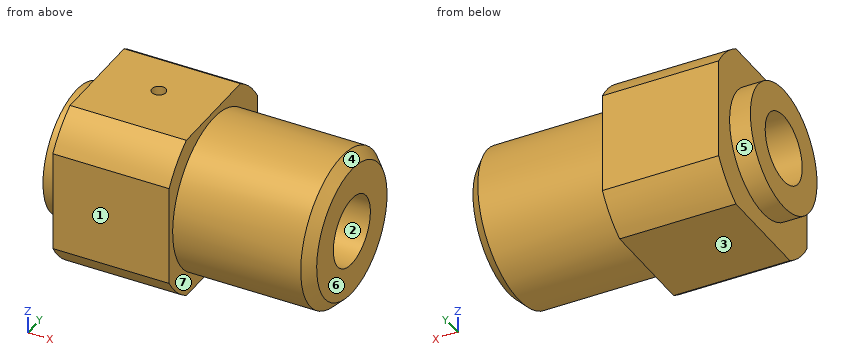
```python
from build123d import *

# Parameters (mm, degrees)
CROQUIS2_OUTSIDE_W      = 40.812
CROQUIS2_OUTSIDE_H      = 40.812
CROQUIS2_OUTSIDE_W_2    = 23.9
CROQUIS2_OUTSIDE_H_2    = 23.9
CORTAR_EXTRUIR1_DEPTH   = 42.788036566
CROQUIS4_R              = 5
CORTAR_EXTRUIR2_DEPTH   = 41.494999691
CROQUIS3_R              = 1
CORTAR_EXTRUIR3_DEPTH   = 13
CROQUIS5_R              = 9
CROQUIS5_R_2            = 5
SALIENTE_EXTRUIR1_DEPTH = 3


with BuildPart() as part:
    # Croquis1 → Revolución1 (revolve)
    with BuildSketch(Plane(origin=(0, 0, 0), x_dir=(1, 0, 0), z_dir=(0, 1, 0)), mode=Mode.PRIVATE) as revoluci_n1_sk:
        Polygon((0, 0), (36.8, 0), (36.8, 9.5), (35.3, 11), (16.8, 11), (16.8, 14), (0, 14), align=None)
    revolve(revoluci_n1_sk.sketch.rotate(Axis((0, 0, 0), (1, 0, 0)), 180), axis=Axis((0, 0, 0), (1, 0, 0)))

    # Croquis2 outside → Cortar-Extruir1 (cut, through all)
    with BuildSketch(Plane(origin=(0, 0, 0), x_dir=(0, 0, -1), z_dir=(1, 0, 0))):
        Rectangle(CROQUIS2_OUTSIDE_W, CROQUIS2_OUTSIDE_H)
        Rectangle(CROQUIS2_OUTSIDE_W_2, CROQUIS2_OUTSIDE_H_2, mode=Mode.SUBTRACT)
    extrude(amount=CORTAR_EXTRUIR1_DEPTH, mode=Mode.SUBTRACT)

    # Croquis4 → Cortar-Extruir2 (cut, through all)
    with BuildSketch(Plane(origin=(36.8, 0, 0), x_dir=(0, 0, -1), z_dir=(1, 0, 0))):
        Circle(CROQUIS4_R)
    extrude(amount=-CORTAR_EXTRUIR2_DEPTH, mode=Mode.SUBTRACT)

    # Croquis3 → Cortar-Extruir3 (cut)
    with BuildSketch(Plane.XY.offset(11.95)):
        with Locations((8.4, 0.993661632)):
            Circle(CROQUIS3_R)
    extrude(amount=-CORTAR_EXTRUIR3_DEPTH, mode=Mode.SUBTRACT)

    # Croquis5 → Saliente-Extruir1 (add)
    with BuildSketch(Plane.ZY):
        with Locations(Location((0, 0, 0), (0, 0, 180))):
            Circle(CROQUIS5_R)
        with Locations(Location((0, 0, 0), (0, 0, 180))):
            Circle(CROQUIS5_R_2, mode=Mode.SUBTRACT)
    extrude(amount=SALIENTE_EXTRUIR1_DEPTH)


solid = part.part
```
Design review of the part built by this model. Coordinates are the model's own, in mm. Face numbers are marked on the shaded views. A direction names the side the tool comes from. Coordinates: 2 decimals unless noted, no trailing zeros. Loops run counter-clockwise (first coordinate to the right, second up) from the corner with the lowest first, then second, coordinate; pieces in that order, holes last. Notation, with made-up numbers: (-16.75, -40) -> (5.25, -40) arc R31 ccw to (5.25, -3) -> close; hole circle Ø5 at (-37.5, 8). An arc over 180 degrees is marked (long way). Answer as a JSON object with one key per item and string values.
Q1. The part is to be moulded in two halves that separate along Y. For the marked faces 1, 2, 3 and 4, say which applies: +Y half, -Y half, draft (parallel to the pull), parting line (faces both ways), or undercut.
Answer block:
{"face 1": "-Y half", "face 2": "undercut", "face 3": "draft", "face 4": "parting line"}
Q2. Take a section at B-B on x = 8.4. Give the boundary of the cut face in (y, z), plus the area to 3 significant figures.
Answer block:
{"outline": "(-11.95, -7.29) arc R14 ccw to (-7.29, -11.95) -> (7.29, -11.95) arc R14 ccw to (11.95, -7.29) -> (11.95, 7.29) arc R14 ccw to (7.29, 11.95) -> (1.99, 11.95) -> (1.99, 4.59) arc R5 cw (long way) to (-0.01, 5) -> (-0.01, 11.95) -> (-7.29, 11.95) arc R14 ccw to (-11.95, 7.29) -> close", "area": "442 mm^2"}
Q3. Tool access review of the marked faces 5, 6 and 7: name each direction out of +Z, -Z, +X, -X, +Y, -Y from which nothing blocks a thin tool from reaching the whole face with its end or side.
Answer block:
{"face 5": "-X", "face 6": "+Z, -Z, +X, +Y, -Y", "face 7": "+X"}
Q4. Take a section at A-A on z = 0. Give the boundary of the cut face in (x, y), plus the area to 3 significant figures.
Answer block:
{"outline": "(-3, -9) -> (0, -9) -> (0, -11.95) -> (16.8, -11.95) -> (16.8, -11) -> (35.3, -11) -> (36.8, -9.5) -> (36.8, -5) -> (-3, -5) -> close; (-3, 5) -> (36.8, 5) -> (36.8, 9.5) -> (35.3, 11) -> (16.8, 11) -> (16.8, 11.95) -> (0, 11.95) -> (0, 9) -> (-3, 9) -> close", "area": "495 mm^2"}
Q5. Take a section at D-D on x = 26. Give the boundary of the cut face in (y, z).
Answer block:
{"outline": "circle Ø22 at (0, 0); hole circle Ø10 at (0, 0)"}
Q6. To check wall thickness, follow L1, parallel to Y at x = 20, z = 0; L2, parallel to Y at x = 11, z = 0; L3, parallel to X at y = 9.5, z = 8.5. State the ranges of each line that lie inside material, in increasing order.
Answer block:
{"L1": "y = -11 to -5, 5 to 11", "L2": "y = -11.95 to -5, 5 to 11.95", "L3": "x = 0 to 16.8"}
Q7. Clearance check with flat-ended pins moving along their axes: pin 1 Ø13 at (y, z) = (0, 0) entering from -X; pin 2 Ø5 at (x, y) = (28, -1) entering from -Z; pin 3 Ø10 at (x, z) = (31, 4.5) entering from -Y; pin 4 Ø6 at (x, y) = (22, 4.5) entering from -Z. State where each tip first meets the part, or that it passes through.
Answer block:
{"pin 1": "stops at x = -3", "pin 2": "stops at z = -11", "pin 3": "stops at y = -11", "pin 4": "stops at z = -10.9"}
Q8. Take a section at C-C on y = 0.5. Give the number of separate pieces and of enclosed holes in the cut face, plus the area to 3 significant figures.
Answer block:
{"separate pieces": "3", "enclosed holes": "0", "area": "485 mm^2"}
